Can you work these out from the model? Positions are in its coordinate system, mm. Face numbers are marked on the shaded views. A direction names the side the tool comes from. Round coordinates to 2 decimals unless told otherwise and drop trailing zeros. Loops run counter-clockwise (first coordinate to the right, second up) from the corner with the lowest first, then second, coordinate; pieces in that order, holes last. Notation, with made-up numbers: M -15,-26.75 L 3,-26.75 A15 cw 3,-18.75 Z; hole C 49,-38 d7. An arc over 180 degrees is marked long. Return JSON: item names as keys, results as strings.
```python
from build123d import *
from OCP.BRepFilletAPI import BRepFilletAPI_MakeChamfer

# Parameters (mm, degrees)
SKETCH1_R                       = 2.5
BOSS_EXTRUDE1_DEPTH             = 10
FILLET1_R                       = 3
CUT_EXTRUDE1_DEPTH              = 19.466185313
FILLET2_R                       = 3
FILLET3_R                       = 3
BOSS_EXTRUDE2_DEPTH             = 3
BOSS_EXTRUDE2_DEPTH_BACK        = 2
SKETCH3_W                       = 7.5
SKETCH3_H                       = 10
BOSS_EXTRUDE3_DEPTH             = 13
BOSS_EXTRUDE3_DIRECTION_2_REACH = 21.339
BOSS_EXTRUDE4_DEPTH             = 5
SKETCH6_R                       = 2.5
CUT_EXTRUDE2_DEPTH              = 87.565417468
FILLET5_R                       = 3
FILLET6_R                       = 1.5
CHAMFER1_SIZE                   = 1
CHAMFER1_SIZE2                  = 0.577350269


with BuildPart() as part:
    # Sketch1 → Boss-Extrude1 (new body)
    with BuildSketch(Plane.XY):
        with BuildLine():
            Line((0, 4), (15, 4))
            Line((15, 4), (15, -4))
            Line((15, -4), (0, -4))
            ThreePointArc((0, -4), (-4, 0), (0, 4))
        make_face()
        Circle(SKETCH1_R, mode=Mode.SUBTRACT)
    extrude(amount=BOSS_EXTRUDE1_DEPTH)

    # Fillet1
    fillet1_edges = [part.edges().sort_by_distance(p)[0] for p in [
        (15, 4, 5),
        (15, -4, 5),
    ]]
    fillet(fillet1_edges, radius=FILLET1_R)

    # Sketch2 → Cut-Extrude1 (cut, through all)
    with BuildSketch(Plane.XY.offset(10)):
        Polygon((15, -1), (0, -4), (15, -4), align=None)
    extrude(amount=-CUT_EXTRUDE1_DEPTH, mode=Mode.SUBTRACT)

    # Fillet2
    # the kernel refuses this fillet: 3 mm, written as the material it takes off along each edge
    with BuildSketch(Plane(origin=(15, -1, -6.055404624), x_dir=(-0.9805806756909201, -0.19611613513818393, 0), z_dir=(0, 0, 1))) as fillet2_piece_1:
        with BuildLine():
            CenterArc((2.42216185, -3), FILLET2_R, 90, 69.740076193)
            Line((-0.39223227, -1.961161351), (-0.448520153, -1.940384578))
            ThreePointArc((-0.448520153, -1.940384578), (-0.254950976, -0.968813708), (-0.058834841, 0.011766968))
            Line((-0.058834841, 0.011766968), (0, 0.06))
            Line((0, 0.06), (2.42216185, 0.06))
            Line((2.42216185, 0.06), (2.42216185, 0))
        make_face()
    extrude(amount=22.110809248, mode=Mode.SUBTRACT)

    # Fillet3
    fillet3_edges = [part.edges().sort_by_distance(p)[0] for p in [
        (0, -4, 5),
    ]]
    fillet(fillet3_edges, radius=FILLET3_R)

    # Sketch3 → Boss-Extrude2 (add, two sides: drawn at the far end of the back side and taken through both)
    with BuildSketch(Plane(origin=(0, 4, 0), x_dir=(1, 0, 0), z_dir=(0, 1, 0)).offset(-BOSS_EXTRUDE2_DEPTH_BACK)):
        with Locations((9.75, -5)):
            Rectangle(SKETCH3_W, SKETCH3_H)
    extrude(amount=BOSS_EXTRUDE2_DEPTH + BOSS_EXTRUDE2_DEPTH_BACK)

    # Sketch4 → Boss-Extrude3 (add)
    with BuildSketch(Plane.XY.offset(10)):
        Polygon((6, 7), (6, 9), (13.5, 9), (13.5, 7), (13.5, 5), (6, 5), align=None)
    extrude(amount=BOSS_EXTRUDE3_DEPTH)

    # Boss-Extrude3 direction 2: up to this face of the body (flat: up to its plane)
    boss_extrude3_direction_2_end = Plane(part.part.faces().sort_by_distance((6.608331714, 1.519169976, 0))[0])
    # Sketch4 → Boss-Extrude3 direction 2 (add, up to the picked face)
    with BuildSketch(Plane.XY.offset(10), mode=Mode.PRIVATE) as boss_extrude3_direction_2_sk1:
        Polygon((6, 7), (6, 9), (13.5, 9), (13.5, 7), (13.5, 5), (6, 5), align=None)
    boss_extrude3_direction_2_tool1 = split(extrude(boss_extrude3_direction_2_sk1.sketch, amount=-BOSS_EXTRUDE3_DIRECTION_2_REACH, mode=Mode.PRIVATE), bisect_by=boss_extrude3_direction_2_end, keep=Keep.BOTH, mode=Mode.PRIVATE)
    add(boss_extrude3_direction_2_tool1.solids().sort_by(Axis((9.75, 7, 10), (0, 0, -1)))[0])

    # Sketch5 → Boss-Extrude4 (add)
    with BuildSketch(Plane.XY.offset(23)):
        with BuildLine():
            Line((13.5, 3.598076211), (13.5, 5))
            Line((13.5, 5), (13.5, 9))
            Line((13.5, 9), (6, 9))
            Line((6, 9), (6, 5))
            Line((6, 5), (6, 4))
            Line((6, 4), (0, 4))
            ThreePointArc((0, 4), (-3.980145848, 0.398044003), (-0.792136593, -3.920780486))
            Line((-0.792136593, -3.920780486), (79.207863407, -3.920780486))
            ThreePointArc((79.207863407, -3.920780486), (82.967291756, -0.161352137), (79.207863407, 3.598076211))
            Line((79.207863407, 3.598076211), (13.5, 3.598076211))
        make_face()
    extrude(amount=BOSS_EXTRUDE4_DEPTH)

    # Sketch6 → Cut-Extrude2 (cut, through all)
    with BuildSketch(Plane(origin=(0, 0, 23), x_dir=(-1, 0, 0), z_dir=(0, 0, -1))):
        with Locations(Location((0, 0, 0), (0, 0, 180))):
            Circle(SKETCH6_R)
        with Locations((-79.207863407, -0.161352137)):
            Circle(SKETCH6_R)
    extrude(amount=-CUT_EXTRUDE2_DEPTH, mode=Mode.SUBTRACT)

    # Fillet5
    # the kernel refuses this fillet: 3 mm, written as the material it adds along each edge
    with BuildSketch(Plane(origin=(13.5, 3.598076211, 23), x_dir=(0, 1, 0), z_dir=(0, 0, 1))) as fillet5_piece_1:
        with BuildLine():
            CenterArc((FILLET5_R, -FILLET5_R), FILLET5_R, 90, 90)
            Line((0, -FILLET5_R), (0, 0))
            Line((0, 0), (FILLET5_R, 0))
        make_face()
    extrude(amount=5)
    with BuildSketch(Plane(origin=(6, 4, 15.5), x_dir=(0, 1, 0), z_dir=(0, 0, 1))) as fillet5_piece_2_section:
        with BuildLine():
            CenterArc((FILLET5_R, FILLET5_R), FILLET5_R, 180, 90)
            Line((0, FILLET5_R), (0, 0))
            Line((0, 0), (FILLET5_R, 0))
        make_face()
    fillet5_piece_2 = extrude(amount=12.5, mode=Mode.PRIVATE)
    fillet5_piece_2 = split(fillet5_piece_2, bisect_by=Plane(origin=(6, 5, 15.5), z_dir=(0, 1, 0)), keep=Keep.TOP, mode=Mode.PRIVATE)
    add(fillet5_piece_2)
    with BuildSketch(Plane(origin=(6, 4, 23), x_dir=(0, 1, 0), z_dir=(0, 0, 1))) as fillet5_piece_3:
        with BuildLine():
            CenterArc((FILLET5_R, FILLET5_R), FILLET5_R, 180, 90)
            Line((0, FILLET5_R), (0, 0))
            Line((0, 0), (FILLET5_R, 0))
        make_face()
    extrude(amount=5)
    with BuildSketch(Plane(origin=(13.5, 3.598076211, 0), x_dir=(0, 1, 0), z_dir=(0, 0, 1))) as fillet5_piece_4:
        with BuildLine():
            CenterArc((1.370550755, -3), FILLET5_R, 90, 41.409622109)
            ThreePointArc((-0.613762728, -0.75), (-0.276396038, -0.399947676), (0, 0))
            Line((0, 0), (1.370550755, 0))
        make_face()
    extrude(amount=10)
    with BuildSketch(Plane(origin=(6, 4, 0), x_dir=(-1, 0, 0), z_dir=(0, 0, 1))) as fillet5_piece_5:
        with BuildLine():
            CenterArc((FILLET5_R, -FILLET5_R), FILLET5_R, 90, 90)
            Line((0, -FILLET5_R), (0, 0))
            Line((0, 0), (FILLET5_R, 0))
        make_face()
    extrude(amount=10)
    with BuildSketch(Plane(origin=(6, 4, -7.5), x_dir=(-1, 0, 0), z_dir=(0, 0, 1))) as fillet5_piece_6_section:
        with BuildLine():
            CenterArc((FILLET5_R, -FILLET5_R), FILLET5_R, 90, 90)
            Line((0, -FILLET5_R), (0, 0))
            Line((0, 0), (FILLET5_R, 0))
        make_face()
    fillet5_piece_6 = extrude(amount=25, mode=Mode.PRIVATE)
    fillet5_piece_6 = split(fillet5_piece_6, bisect_by=Plane(origin=(6, 4, 10), z_dir=(0, 0, 1)), keep=Keep.TOP, mode=Mode.PRIVATE)
    fillet5_piece_6 = split(fillet5_piece_6, bisect_by=Plane(origin=(6, 5, -7.5), z_dir=(0, 1, 0)), keep=Keep.TOP, mode=Mode.PRIVATE)
    add(fillet5_piece_6)

    # Fillet6
    fillet6_edges = [part.edges().sort_by_distance(p)[0] for p in [
        (6, 9, 14),
        (13.5, 9, 14),
    ]]
    fillet(fillet6_edges, radius=FILLET6_R)

    # Chamfer1: one chamfer whose edges measure the first distance from different faces: ONE call of the kernel's chamfer builder (chamfer() names one face for all edges)
    chamfer1_edges_1 = [part.edges().sort_by_distance(p)[0] for p in [
        (47.853931704, 3.598076211, 28),
    ]]
    chamfer1_side_1 = [part.faces().sort_by_distance(p)[0] for p in [
        (47.853931704, 3.598076211, 25.5),
    ]]
    chamfer1_edges_2 = [part.edges().sort_by_distance(p)[0] for p in [
        (-3.980145848, 0.398044003, 28),
    ]]
    chamfer1_side_2 = [part.faces().sort_by_distance(p)[0] for p in [
        (-3.980145848, 0.398044003, 25.5),
    ]]
    chamfer1_edges_3 = [part.edges().sort_by_distance(p)[0] for p in [
        (39.207863407, -3.920780486, 28),
    ]]
    chamfer1_side_3 = [part.faces().sort_by_distance(p)[0] for p in [
        (39.207863407, -3.920780486, 25.5),
    ]]
    chamfer1_edges_4 = [part.edges().sort_by_distance(p)[0] for p in [
        (82.967291756, -0.161352137, 28),
    ]]
    chamfer1_side_4 = [part.faces().sort_by_distance(p)[0] for p in [
        (82.967291756, -0.161352137, 25.5),
    ]]
    chamfer1_edges_5 = [part.edges().sort_by_distance(p)[0] for p in [
        (13.5, 7.049038106, 28),
    ]]
    chamfer1_side_5 = [part.faces().sort_by_distance(p)[0] for p in [
        (13.5, 6.301445777, 12.480297412),
    ]]
    chamfer1_edges_6 = [part.edges().sort_by_distance(p)[0] for p in [
        (1.5, 4, 28),
    ]]
    chamfer1_side_6 = [part.faces().sort_by_distance(p)[0] for p in [
        (1.5, 4, 25.5),
    ]]
    chamfer1_edges_7 = [part.edges().sort_by_distance(p)[0] for p in [
        (14.378679656, 4.476755868, 28),
    ]]
    chamfer1_side_7 = [part.faces().sort_by_distance(p)[0] for p in [
        (14.378679656, 4.476755868, 25.5),
    ]]
    chamfer1_edges_8 = [part.edges().sort_by_distance(p)[0] for p in [
        (5.121320344, 4.878679656, 28),
    ]]
    chamfer1_side_8 = [part.faces().sort_by_distance(p)[0] for p in [
        (5.121320344, 4.878679656, 14),
    ]]
    chamfer1_edges_9 = [part.edges().sort_by_distance(p)[0] for p in [
        (9.75, 9, 28),
    ]]
    chamfer1_side_9 = [part.faces().sort_by_distance(p)[0] for p in [
        (9.75, 9, 14),
    ]]
    chamfer1_edges_10 = [part.edges().sort_by_distance(p)[0] for p in [
        (6, 7.25, 28),
    ]]
    chamfer1_side_10 = [part.faces().sort_by_distance(p)[0] for p in [
        (6, 7.25, 14),
    ]]
    chamfer1_edges_11 = [part.edges().sort_by_distance(p)[0] for p in [
        (13.060660172, 8.560660172, 28),
    ]]
    chamfer1_side_11 = [part.faces().sort_by_distance(p)[0] for p in [
        (13.060660172, 8.560660172, 14),
    ]]
    chamfer1_edges_12 = [part.edges().sort_by_distance(p)[0] for p in [
        (6.439339828, 8.560660172, 28),
    ]]
    chamfer1_side_12 = [part.faces().sort_by_distance(p)[0] for p in [
        (6.439339828, 8.560660172, 14),
    ]]
    chamfer1 = BRepFilletAPI_MakeChamfer(part.part.solid().wrapped)
    for e in chamfer1_edges_1:
        chamfer1.Add(CHAMFER1_SIZE, CHAMFER1_SIZE2, e.wrapped, chamfer1_side_1[0].wrapped)  # the first distance lies on this face
    for e in chamfer1_edges_2:
        chamfer1.Add(CHAMFER1_SIZE, CHAMFER1_SIZE2, e.wrapped, chamfer1_side_2[0].wrapped)  # the first distance lies on this face
    for e in chamfer1_edges_3:
        chamfer1.Add(CHAMFER1_SIZE, CHAMFER1_SIZE2, e.wrapped, chamfer1_side_3[0].wrapped)  # the first distance lies on this face
    for e in chamfer1_edges_4:
        chamfer1.Add(CHAMFER1_SIZE, CHAMFER1_SIZE2, e.wrapped, chamfer1_side_4[0].wrapped)  # the first distance lies on this face
    for e in chamfer1_edges_5:
        chamfer1.Add(CHAMFER1_SIZE, CHAMFER1_SIZE2, e.wrapped, chamfer1_side_5[0].wrapped)  # the first distance lies on this face
    for e in chamfer1_edges_6:
        chamfer1.Add(CHAMFER1_SIZE, CHAMFER1_SIZE2, e.wrapped, chamfer1_side_6[0].wrapped)  # the first distance lies on this face
    for e in chamfer1_edges_7:
        chamfer1.Add(CHAMFER1_SIZE, CHAMFER1_SIZE2, e.wrapped, chamfer1_side_7[0].wrapped)  # the first distance lies on this face
    for e in chamfer1_edges_8:
        chamfer1.Add(CHAMFER1_SIZE, CHAMFER1_SIZE2, e.wrapped, chamfer1_side_8[0].wrapped)  # the first distance lies on this face
    for e in chamfer1_edges_9:
        chamfer1.Add(CHAMFER1_SIZE, CHAMFER1_SIZE2, e.wrapped, chamfer1_side_9[0].wrapped)  # the first distance lies on this face
    for e in chamfer1_edges_10:
        chamfer1.Add(CHAMFER1_SIZE, CHAMFER1_SIZE2, e.wrapped, chamfer1_side_10[0].wrapped)  # the first distance lies on this face
    for e in chamfer1_edges_11:
        chamfer1.Add(CHAMFER1_SIZE, CHAMFER1_SIZE2, e.wrapped, chamfer1_side_11[0].wrapped)  # the first distance lies on this face
    for e in chamfer1_edges_12:
        chamfer1.Add(CHAMFER1_SIZE, CHAMFER1_SIZE2, e.wrapped, chamfer1_side_12[0].wrapped)  # the first distance lies on this face
    add(Compound.cast(chamfer1.Shape()), mode=Mode.REPLACE)


solid = part.part
```
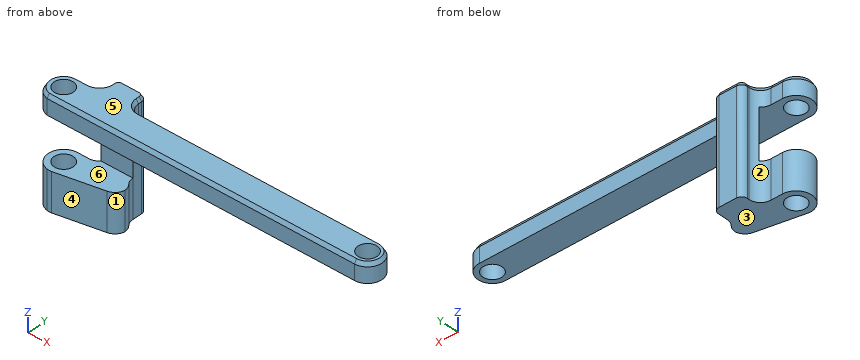
Q1. Thinking about a two-plate mould opening in Z: for the marked faces 3, 4, 5 and 6, which applies, pulls with the +Z half, pulls with the -Z half, needs draft (parallel to the pull), parting line crosses it, or undercut?
Results:
{"face 3": "pulls with the -Z half", "face 4": "needs draft", "face 5": "pulls with the +Z half", "face 6": "undercut"}
Q2. If I drill on line 1 along Y through (x, z) = (0, 2.75); line 2 along X through (y, z) = (-0.5, 26); line 3 along Y through (x, z) = (40.5, 23.25), over which ranges is the centre line in solid material (lowest first)?
Results:
{"line 1": "y = -3.97 to -2.5, 2.5 to 4", "line 2": "x = -3.97 to -2.45, 2.45 to 76.73, 81.68 to 82.95", "line 3": "y = -3.92 to 3.6"}
Q3. Suppose I cut it at C-C, the plane x = 51. Please give me the cut outline in (y, z), plus the area to 3 significant figures.
Results:
{"outline": "M -3.92,23 L 3.6,23 L 3.6,27 L 3.02,28 L -3.34,28 L -3.92,27 Z", "area": "37.0 mm2"}
Q4. Suppose I cut it at B-B, the plane z = 12. Please give me the cut outline in (x, y), plus the area to 3 significant figures.
Results:
{"outline": "M 5.24,5 L 13.5,5 L 13.5,7.5 A1.5 ccw 12,9 L 7.5,9 A1.5 ccw 6,7.5 L 6,7 A3 cw Z", "area": "29.5 mm2"}
Q5. On a 3-axis mill with a long thin cutter (end or side, diameter ignored), from which of +Z, -Z, +X, -X, +Y, -Y can I reach the whole of each face in a straight line? I mean the marked faces 1 and 2. Say none if no direction works.
Results:
{"face 1": "-Z, +X, -Y", "face 2": "+Z, -Z, -X, +Y"}
Q6. Suppose I cut it at A-A, the plane z = 8. Please give me the cut outline in (x, y), plus the area to 3 significant figures.
Results:
{"outline": "M -0.79,-3.92 A3 ccw 0.39,-3.92 L 12.62,-1.48 A3 ccw 15,1 A3 ccw 14.25,2.98 A3 cw 13.5,4.97 L 13.5,7.5 A1.5 ccw 12,9 L 7.5,9 A1.5 ccw 6,7.5 L 6,7 A3 cw 3,4 L 0,4 A4 ccw Z; hole C 0,0 d5", "area": "139 mm2"}
Q7. I'm going to push flat-ended pins straight in: pin 1 Ø6 at (x, y) = (37.5, 7.5) entering from +Z; pin 2 Ø3 at (x, z) = (63, 25) entering from +Y; pin 3 Ø3.5 at (x, z) = (1.5, 24) entering from +Y; pin 4 Ø4 at (x, z) = (51, 24) entering from -Y. Where does each tip first touch, or does it pass through?
Results:
{"pin 1": "passes through", "pin 2": "stops at y = 3.6", "pin 3": "stops at y = 4.01", "pin 4": "stops at y = -3.92"}
